Input: part model. Units: mm. Frame: model coordinates. Round coordinates to 2 decimals unless told otherwise and drop trailing zeros. Write each loop counter-clockwise with the first axis right and the second up, starting at its lowest first coordinate (ties: lowest second). Pieces come first, ordered by that corner, then holes. Notation, with made-up numbers: M 79,13.5 L 85,13.5 A33 cw 85,45.5 Z; hole C 6.25,73.5 d10. An arc over 180 degrees is marked long. Use one line per item in the form item = value. Start each with the question number.
Autodesk Fusion 360 part; units mm, degrees
sketch "Sketch1" plane through (0, 0, 0) normal (0, 1, 0) x (1, 0, 0)
  circle A0 centre (0, 0) radius 8
  circle A1 centre (0, 0) radius 6.5
  dimension "d1" = 16
  dimension "d2" = 13
extrude "Extrude1" add sketch "Sketch1" along normal mid plane 22
chamfer "Chamfer1" distance 0.2 angle 45 2 edges at (-7.4586, 11, 2.8929) (-7.4586, -11, -2.8929)
Item 1: Cut plane C-C (y = -9.5). Output: boundary loops of the cut face in (x, z).
Item 2: Cut plane B-B (x = 0). Output: boundary loops of the cut face in (y, z), plus the area to 3 significant figures.
Item 3: First-contact query: pin 1 (8 mm diameter, centred on x = 4.5, y = -8, fed in from -Z); pin 2 (3 mm diameter, centred on x = 3, y = -3.5, fed in from +Z); pin 3 (6 mm diameter, centred on y = -6.5, z = -3.5, fed in from +X). Flat tips, straight axial feed; report the tip coordinate or a pass-through.
Item 4: Cut plane A-A (z = 0). Output: boundary loops of the cut face in (x, y), plus the area to 3 significant figures.
Item 5: Draft query along Z for faces 1 (the face through (-3, 11, -6)), 2 (the face through (-1.73, -0.15, -7.81)), 3 (the face through (-5.158, 0.154, 3.955)). Return one class per face: +Z half, -Z half, draft (parallel to the pull), parting line (faces both ways), or undercut.
Item 6: Ray query, line 1 (Z direction, x = 0, y = 0); line 2 (Z direction, x = 3.75, y = -3.75). Return the intervals inside material, ascending. Write a range as from..to.
Final values:
q1.outline = C 0,0 d16; hole C 0,0 d13
q2.outline = M -11,-7.8 L -10.8,-8 L 10.8,-8 L 11,-7.8 L 11,-6.5 L -11,-6.5 Z; M -11,6.5 L 11,6.5 L 11,7.8 L 10.8,8 L -10.8,8 L -11,7.8 Z
q2.area = 65.9 mm^2
q3.pin_1 = -7.98
q3.pin_2 = 7.86
q3.pin_3 = 7.98
q4.outline = M -8,-10.8 L -7.8,-11 L -6.5,-11 L -6.5,11 L -7.8,11 L -8,10.8 Z; M 6.5,-11 L 7.8,-11 L 8,-10.8 L 8,10.8 L 7.8,11 L 6.5,11 Z
q4.area = 65.9 mm^2
q5.face_1 = draft
q5.face_2 = parting line
q5.face_3 = undercut
q6.line_1 = -8..-6.5, 6.5..8
q6.line_2 = -7.07..-5.31, 5.31..7.07
